Can you work these out from the model? Positions are in its coordinate system, mm. A direction names the side the tool comes from. Round coordinates to 2 decimals unless told otherwise and drop trailing zeros. Write each loop counter-clockwise with the first axis right and the second up, starting at its lowest first coordinate (ties: lowest second). Pieces come first, ordered by that corner, then holes. Notation, with made-up numbers: M 46.25,-4.5 L 98.25,-4.5 A24 cw 98.25,7.5 Z; hole C -2,7.5 d4. An arc over 180 degrees is marked long. Answer as a JSON object with one key per item and string values. Group by question number.
1) On a 3-axis mill with a long thin cutter (end or side, diameter ignored), from which of +Z, -Z, +X, -X, +Y, -Y can I reach the whole of each face in a straight line? I mean faces 4 (the flat face through (0, -12, 130)), 5 (the cylindrical face through (-13.289, 13.196, 157.837)). Say none if no direction works.
2) If we mould it in two halves opening along X, with no side actions, what happens to faces 1 (the flat face through (0, 12, 130)), 2 (the cylindrical face through (13.289, -13.196, 103.803)), 3 (the flat face through (-12.85, -0.21, 243.84))? For each: +X half, -X half, draft (parallel to the pull), parting line (faces both ways), or undercut.
3) Suppose I cut it at C-C, the plane z = 141. Write out the boundary of the cut face in (x, y), and give its area (3 significant figures).
4) Suppose I cut it at A-A, the plane y = -5.5. Write out the boundary of the cut face in (x, z).
5) Please list where these lines run through material, in increasing order: L1, parallel to X at y = -4.75, z = 123; L2, parallel to Y at x = -11, z = 134. Write a range as [from, to].
6) I'm going to push flat-ended pins straight in: pin 1 Ø2 at (x, y) = (-10.5, -2) entering from -Z; pin 2 Ø9 at (y, z) = (-1.5, 67.5) entering from -X; pin 3 Ø1 at (y, z) = (11, 150.5) entering from -X; pin 4 Ø1.5 at (y, z) = (-10.5, 171.5) entering from +X. Where does each tip first touch, or does it pass through?
7) Suppose I cut it at D-D, the plane z = 196. Write out the boundary of the cut face in (x, y), and give its area (3 significant figures).
8) Suppose I cut it at B-B, the plane x = -6. Write out the boundary of the cut face in (y, z).
Autodesk Inventor part; units mm, degrees
ref_plane "Start Plane" through (0, 0, 19.0301) normal (0, 0, 1) x (1, 0, 0)
ref_plane "End Plane" through (0, 0, 245.0248) normal (0, 0, 1) x (1, 0, 0)
ref_plane "Work Plane4" through (-108.1214, 9, 364.6022) normal (-0.9468, 0, -0.3219) x (-0.3219, 0, 0.9468)
ref_plane "Start Plane" through (0, 0, 19.0301) normal (0, 0, 1) x (1, 0, 0)
ref_plane "End Plane" through (0, 0, 245.0248) normal (0, 0, 1) x (1, 0, 0)
sketch "Sketch" plane through (0, 0, 0) normal (0, 0, 1) x (1, 0, 0)
  line L0 (-15, -9) -> (-15, 9)
  line L1 (-9, 15) -> (9, 15)
  line L2 (15, 9) -> (15, -9)
  line L3 (9, -15) -> (-9, -15)
  arc A0 (-15, -9) -> (-9, -15) centre (-9, -9) ccw
  arc A1 (-9, 15) -> (-15, 9) centre (-9, 9) ccw
  arc A2 (15, 9) -> (9, 15) centre (9, 9) ccw
  arc A3 (9, -15) -> (15, -9) centre (9, -9) ccw
  arc A4 (-9, 12) -> (-12, 9) centre (-9, 9) ccw
  line L4 (-9, 12) -> (9, 12)
  arc A5 (12, 9) -> (9, 12) centre (9, 9) ccw
  line L5 (12, 9) -> (12, -9)
  arc A6 (9, -12) -> (12, -9) centre (9, -9) ccw
  line L6 (9, -12) -> (-9, -12)
  arc A7 (-12, -9) -> (-9, -12) centre (-9, -9) ccw
  line L7 (-12, -9) -> (-12, 9)
  line L8 (0, 22.7397) -> (0, -22.7397) construction
  line L9 (-22.7397, 0) -> (22.7397, 0) construction
  dimension "d7" = 6
  dimension "d10" = 30
  dimension "d11" = 30
  dimension "d12" = 3
  dimension "d15" = 15
  dimension "d16" = 15
extrude "Body" add sketch "Sketch" along normal up to surface (225.9947 mm away) from surface at 19.0301
sketch "Sketch3" plane through (0, 0, 0) normal (0, 0, 1) x (1, 0, 0)
  line L0 (0, 0) -> (10, 0)
ref_plane "Work Plane3" through (0, 0, 0) normal (0, -1, 0) x (1, 0, 0)
ref_plane "Work Plane4" through (-108.1214, 9, 364.6022) normal (-0.9468, 0, -0.3219) x (-0.3219, 0, 0.9468)
split "Split1" plane through (-108.1214, 9, 364.6022) removes the side toward (-0.9468, 0, -0.3219)
ref_plane "Work Plane5" through (75.6471, 9, 41.5633) normal (0.3219, 0, -0.9468) x (-0.9468, 0, -0.3219)
split "Split2" plane through (75.6471, 9, 41.5633) removes the side toward (0.3219, 0, -0.9468)
ref_plane "Work Plane6" through (-14.2016, 9, 259.2264) normal (0.9468, 0, 0.3219) x (0.3219, 0, -0.9468)
split "Split3" plane through (-14.2016, 9, 259.2264) removes the side toward (0.9468, 0, 0.3219)
ref_plane "Work Plane7" through (-75.6471, 9, 222.4916) normal (-0.3219, 0, 0.9468) x (0.9468, 0, 0.3219)
split "Split4" plane through (-75.6471, 9, 222.4916) removes the side toward (-0.3219, 0, 0.9468)
sketch "Sketch4" plane through (0, 0, 0) normal (0, -1, 0) x (1, 0, 0)
  line L0 (-2, 19.0301) -> (12, 19.0301)
  line L1 (-2, 245.0248) -> (12, 245.0248)
  dimension "d18" = 225.9947
equation "\"d7\" = G_IR"
equation "\"d10\" = G_H"
equation "\"d11\" = G_W"
equation "\"d12\" = G_T"
equation "\"d15\" = 0.5 * d10"
equation "\"d16\" = 0.5 * d11"
equation "\"d3\" = G_L"
equation "\"G_W\" = 30"
equation "\"G_H\" = 30"
equation "\"G_T\" = 3"
equation "\"G_IR\" = 6"
equation "\"G_L\" = d18"
equation "\"G_OFFSET_START\" = -19.03013"
equation "\"G_OFFSET_END\" = -19.03013"
equation "\"d13\" = -G_OFFSET_START"
equation "\"d14\" = G_OFFSET_END + B_L"
equation "\"B_L\" = 264.05492"
properties part number "DIN EN 10219-2 - 30 x 30 x 3  - 225.99" material "Steel, Mild"
Results:
{
 "1": {"face 4": "+Z, -Z", "face 5": "+Z, -Z, -X, +Y"},
 "2": {"face 1": "undercut", "face 2": "+X half", "face 3": "-X half"},
 "3": {"outline": "M -15,-9 A6 ccw -9,-15 L 9,-15 A6 ccw 15,-9 L 15,9 A6 ccw 9,15 L -9,15 A6 ccw -15,9 Z; hole M -12,-9 A3 ccw -9,-12 L 9,-12 A3 ccw 12,-9 L 12,9 A3 ccw 9,12 L -9,12 A3 ccw -12,9 Z", "area": "301 mm^2"},
 "4": {"outline": "M -15,90.71 L -12,81.88 L -12,244.13 L -15,243.11 Z; M 12,19.92 L 15,20.94 L 15,173.34 L 12,182.16 Z"},
 "5": {"L1": "[-15, -12], [12, 15]", "L2": "[-14.66, -11.24], [11.24, 14.66]"},
 "6": {"pin 1": "through", "pin 2": "x = 12", "pin 3": "x = -14.81", "pin 4": "x = 14.95"},
 "7": {"outline": "M -15,-9 A6 ccw -9,-15 L 7.29,-15 L 7.29,-12 L -9,-12 A3 cw -12,-9 L -12,9 A3 cw -9,12 L 7.29,12 L 7.29,15 L -9,15 A6 ccw -15,9 Z", "area": "194 mm^2"},
 "8": {"outline": "M -15,64.23 L -12,64.23 L -12,235.1 L -15,235.1 Z; M 12,64.23 L 15,64.23 L 15,235.1 L 12,235.1 Z"}
}
